Design review of the part built by this model. Coordinates are the model's own, in mm. Face numbers are marked on the shaded views. A direction names the side the tool comes from. Round coordinates to 2 decimals unless told otherwise and drop trailing zeros. Loops run counter-clockwise (first coordinate to the right, second up) from the corner with the lowest first, then second, coordinate; pieces in that order, holes last. Notation, with made-up numbers: M 79.5,-17 L 110.5,-17 A13 ccw 110.5,-12 Z; hole C 83,45 d9. An arc over 180 degrees is marked long. One line per item, written item: value. Start each with the question number.
Item 1: We need section C-C (y = -0.3). Write out the cut boundary in (x, z), then the cut area to 3 significant figures.
Item 2: For the marked faces 1, 2, 3 and 4, list the 3-axis set-ups (+Z, -Z, +X, -X, +Y, -Y) from which the entire face can be reached by the end or side of a thin tool; tool diameter is ignored.
Item 3: We need section B-B (z = -0.75). Write out the cut boundary in (x, y) (3 decimals), then the cut area to 3 significant figures.
Item 4: For line 1 along X through (y, z) = (1.45, 2.75); line 2 along X through (y, z) = (2.05, -3); line 3 along Y through (x, z) = (-0.75, -1.25), list the stretches that pass through material, from the lowest coordinate up.
from build123d import *

# Parameters (mm, degrees)
SKETCH1_R                = 3.556
BOSS_EXTRUDE1_DEPTH      = 3.175
SKETCH2_R                = 2.38125
BOSS_EXTRUDE2_DEPTH      = 0.127
CUT_EXTRUDE3_DEPTH       = 6.947343693
FILLET1_R                = 0.1016
CIRPATTERN3_COUNT        = 15
FILLET1_OF_CIRPATTERN3_R = 0.1016
SKETCH5_R                = 0.8509
CUT_EXTRUDE2_DEPTH       = 3.302
SKETCH6_R                = 0.1905
BOSS_EXTRUDE3_DEPTH      = 1.905
CIRPATTERN2_COUNT        = 3


with BuildPart() as part:
    # Sketch1 → Boss-Extrude1 (new body)
    with BuildSketch(Plane(origin=(0, 0, 0), x_dir=(1, 0, 0), z_dir=(0, 1, 0))):
        with Locations(Location((0, 0, 0), (0, 0, 270))):
            Circle(SKETCH1_R)
    extrude(amount=BOSS_EXTRUDE1_DEPTH)

    # Sketch2 → Boss-Extrude2 (add)
    with BuildSketch(Plane(origin=(0, 3.175, 0), x_dir=(1, 0, 0), z_dir=(0, 1, 0))):
        with Locations(Location((0, 0, 0), (0, 0, 270))):
            Circle(SKETCH2_R)
    extrude(amount=BOSS_EXTRUDE2_DEPTH)

    # Sketch8 → Cut-Extrude3 (cut, through all)
    with BuildSketch(Plane(origin=(0, 3.175, 0), x_dir=(1, 0, 0), z_dir=(0, 1, 0))):
        with BuildLine():
            Line((-0.273921569, 2.780540051), (-0.254, 2.578318956))
            ThreePointArc((-0.254, 2.578318956), (0, 2.5908), (0.254, 2.578318956))
            Line((0.254, 2.578318956), (0.273921569, 2.780540051))
            ThreePointArc((0.273921569, 2.780540051), (0.38769625, 3.17325346), (0.635, 3.498844238))
            ThreePointArc((0.635, 3.498844238), (0, 3.556), (-0.635, 3.498844238))
            ThreePointArc((-0.635, 3.498844238), (-0.38769625, 3.17325346), (-0.273921569, 2.780540051))
        make_face()
    cut_extrude3 = extrude(amount=-CUT_EXTRUDE3_DEPTH, mode=Mode.SUBTRACT)

    # Fillet1
    fillet1_edges = [part.edges().sort_by_distance(p)[0] for p in [
        (0.254, 1.5875, -2.578318956),
        (-0.254, 1.5875, -2.578318956),
    ]]
    fillet(fillet1_edges, radius=FILLET1_R)

    # CirPattern3: Cut-Extrude3 ×15 about axis
    cirpattern3_axis = Axis((0, 0, 0), (0, 1, 0))
    for i in range(1, CIRPATTERN3_COUNT):
        add(cut_extrude3.rotate(cirpattern3_axis, i * 360 / CIRPATTERN3_COUNT), mode=Mode.SUBTRACT)

    # Fillet1 of CirPattern3
    fillet1_of_cirpattern3_edges = [part.edges().sort_by_distance(p)[0] for p in [
        (-0.816656251, 1.5875, -2.458722678),
        (-1.280737343, 1.5875, -2.252100463),
        (-1.746105217, 1.5875, -1.913990912),
        (-2.086023565, 1.5875, -1.536473341),
        (-2.373636728, 1.5875, -1.03831273),
        (-2.530617361, 1.5875, -0.555176019),
        (-2.590744885, 1.5875, 0.016899157),
        (-2.537644426, 1.5875, 0.52211628),
        (-2.359889715, 1.5875, 1.069189026),
        (-2.105889715, 1.5875, 1.509129931),
        (-1.720988175, 1.5875, 1.936606398),
        (-1.310007542, 1.5875, 2.235201307),
        (-0.784512144, 1.5875, 2.469166931),
        (-0.287613163, 1.5875, 2.57478607),
        (0.287613163, 1.5875, 2.57478607),
        (0.784512144, 1.5875, 2.469166931),
        (1.310007542, 1.5875, 2.235201307),
        (1.720988175, 1.5875, 1.936606398),
        (2.105889715, 1.5875, 1.509129931),
        (2.359889715, 1.5875, 1.069189026),
        (2.537644426, 1.5875, 0.52211628),
        (2.590744885, 1.5875, 0.016899157),
        (2.530617361, 1.5875, -0.555176019),
        (2.373636728, 1.5875, -1.03831273),
        (2.086023565, 1.5875, -1.536473341),
        (1.746105217, 1.5875, -1.913990912),
        (1.280737343, 1.5875, -2.252100463),
        (0.816656251, 1.5875, -2.458722678),
    ]]
    fillet(fillet1_of_cirpattern3_edges, radius=FILLET1_OF_CIRPATTERN3_R)

    # Sketch5 → Cut-Extrude2 (cut)
    with BuildSketch(Plane.XZ):
        with Locations(Location((0, 0, 0), (0, 0, 270))):
            Circle(SKETCH5_R)
    extrude(amount=-CUT_EXTRUDE2_DEPTH, mode=Mode.SUBTRACT)

    # Sketch6 → Boss-Extrude3 (add)
    with BuildSketch(Plane.XZ):
        with Locations(Location((0, -1.778, 0), (0, 0, 90))):
            Circle(SKETCH6_R)
    boss_extrude3 = extrude(amount=BOSS_EXTRUDE3_DEPTH)

    # CirPattern2: Boss-Extrude3 ×3 about axis
    cirpattern2_axis = Axis((0, 0, 0), (0, 1, 0))
    for i in range(1, CIRPATTERN2_COUNT):
        add(boss_extrude3.rotate(cirpattern2_axis, i * 360 / CIRPATTERN2_COUNT))


solid = part.part
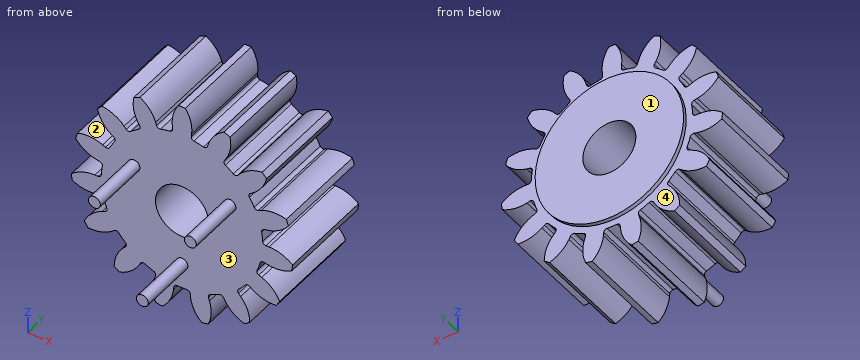
A:
1. outline: C -1.54,0.89 d0.38; C 0,-1.78 d0.38; C 1.54,0.89 d0.38
1. area: 0.342 mm2
2. face 1: +Z, -Z, +X, -X, +Y
2. face 2: +Y, -Y
2. face 3: -Y
2. face 4: +Y
3. outline: M -2.48,0 L -0.402,0 L -0.402,3.302 L -2.26,3.302 L -2.26,3.175 L -2.48,3.175 Z; M 0.402,0 L 2.48,0 L 2.48,3.175 L 2.26,3.175 L 2.26,3.302 L 0.402,3.302 Z
3. area: 13.7 mm2
4. line 1: -1.54 to -0.88, -0.31 to 0.31, 0.88 to 1.54
4. line 2: -0.94 to -0.32, 0.32 to 0.94
4. line 3: 0 to 3.3
